Autodesk Inventor part; units mm, degrees
ref_plane "Płaszczyzna konstrukcyjna1" through (26, 10.6066, 10.6066) normal (0, 0.7071, 0.7071) x (-1, 0, 0)
ref_plane "Płaszczyzna konstrukcyjna2" through (26, 10.6066, -10.6066) normal (0, 0.7071, -0.7071) x (-1, 0, 0)
ref_plane "YZ Plane" through (0, 0, 0) normal (1, 0, 0) x (0, 1, 0)
sketch "Szkic1" plane through (0, 0, 0) normal (1, 0, 0) x (0, 1, 0)
  circle A0 centre (0, 0) radius 15
  dimension "d0" = 30
extrude "Wyciągnięcie proste1" add sketch "Szkic1" along normal blind 26
sketch "Szkic2" plane through (26, 0, 0) normal (1, 0, 0) x (0, 0, -1)
  point P0 (0, 0)
  point P1 (0, 0)
hole "Otwór1" at (26, 0, 0) direction (-1, 0, 0) diameter 8.5 end through all
sketch "Szkic3" plane through (26, 0, 0) normal (1, 0, 0) x (0, 0, -1)
  point P0 (0, 0)
  point P1 (11, 0)
  point P2 (0, 11)
  point P3 (-11, 0)
  point P4 (0, -11)
  dimension "d10" = 11
  dimension "d13" = 360
hole "Otwór2" at (26, 0, -11) at (26, 11, 0) at (26, 0, 11) at (26, -11, 0) direction (-1, 0, 0) diameter 3.5 depth 26 tip angle 118
sketch "Szkic4" plane through (26, 0, 0) normal (1, 0, 0) x (0, 0, -1)
  line L0 (0, 0) -> (-10.6066, 10.6066)
  line L1 (0, 0) -> (15, 0) construction
  line L2 (0, 0) -> (10.6066, 10.6066)
  line L3 (0, 0) -> (15, 0) construction
  dimension "d22" = 15
  dimension "d23" = 135
  dimension "d24" = 15
  dimension "d25" = 45
ref_plane "Płaszczyzna konstrukcyjna1" through (26, 10.6066, 10.6066) normal (0, 0.7071, 0.7071) x (-1, 0, 0)
ref_plane "Płaszczyzna konstrukcyjna2" through (26, 10.6066, -10.6066) normal (0, 0.7071, -0.7071) x (-1, 0, 0)
sketch "Szkic7" plane through (0, 0, 0) normal (-1, 0, 0) x (0, 0, 1)
  circle A0 centre (0, 0) radius 6.5
  dimension "d42" = 13
extrude "Wyciągnięcie proste2" cut sketch "Szkic7" against normal blind 5
sketch "Szkic13" plane through (5, 0, 0) normal (-1, 0, 0) x (0, 0, 1)
  circle A0 centre (0, 0) radius 5.5
  dimension "d80" = 11
extrude "Wyciągnięcie proste5" cut sketch "Szkic13" against normal blind 0.5
sketch "Szkic14" plane through (26, 0, 0) normal (1, 0, 0) x (0, 0, -1)
  circle A0 centre (0, 0) radius 6.5
  dimension "d83" = 13
extrude "Wyciągnięcie proste6" cut sketch "Szkic14" against normal blind 5
sketch "Szkic15" plane through (21, 0, 0) normal (1, 0, 0) x (0, 0, -1)
  circle A0 centre (0, 0) radius 5.5
  dimension "d86" = 11
extrude "Wyciągnięcie proste7" cut sketch "Szkic15" against normal blind 0.5
equation "\"d0\" = radius"
equation "\"d16\" = d1"
equation "\"d20\" = d1"
equation "\"d22\" = 0.5 * radius"
equation "\"d24\" = d22"
equation "\"radius\" = 30"
properties part number "piasta_kola_przedniego_fi8" material "Aluminum 6061"
Work out the finished part from the listing and answer in its coordinate system (mm). A direction names the side the tool comes from. Round coordinates to 2 decimals unless told otherwise and drop trailing zeros. Write each loop counter-clockwise with the first axis right and the second up, starting at its lowest first coordinate (ties: lowest second). Pieces come first, ordered by that corner, then holes. Notation, with made-up numbers: (2, -36.5) -> (28, -36.5) arc R5 ccw to (28, -29.5) -> close; hole circle Ø8 at (-27, -31). An arc over 180 degrees is marked (long way). Write each question's results on one line, items separated by ' | '.
Q1. Determine the mould class of faces 1 (the cylindrical face through (2.465, -3.955, -5.158)), 2 (the flat face through (0, 6, -3)), 3 (the cylindrical face through (12.818, -14.985, -0.66)), 4 (the cylindrical face through (20.75, -5.37, 1.19)) for opening direction Y: released by +Y, released by -Y, zero draft, split by the parting line, or undercut.
Data:
face 1: undercut | face 2: zero draft | face 3: split by the parting line | face 4: undercut
Q2. Section D-D, the plane x = 6.75 is taken. Write down the section's boundary in (y, z).
Data:
outline: circle Ø30 at (0, 0); hole circle Ø3.5 at (-11, 0); hole circle Ø8.5 at (0, 0); hole circle Ø3.5 at (0, -11); hole circle Ø3.5 at (0, 11); hole circle Ø3.5 at (11, 0)
Q3. Section C-C, the plane y = 11 is taken. Write down the section's boundary in (x, z).
Data:
outline: (0, -10.2) -> (26, -10.2) -> (26, -1.75) -> (0, -1.75) -> close; (0, 1.75) -> (26, 1.75) -> (26, 10.2) -> (0, 10.2) -> close
Q4. Flat-ended cylindrical pins translate along their axes: P1, Ø9, axis at y = 0, z = 0, coming from the -X side; P2, Ø10, axis at x = 7, z = -11.5, coming from the +Y side; P3, Ø12, axis at x = 20, z = 8.5, coming from the +Y side. Find the tip coordinate at first contact, or state that the pin passes through.
Data:
P1: x = 5.5 | P2: y = 13.52 | P3: y = 14.79
Q5. Which of the six approach directions +Z, -Z, +X, -X, +Y, -Y give full straight-line access (tool end or side, diameter ignored) to faces 5 (the cylindrical face through (23.535, -3.955, 5.158)), 6 (the cylindrical face through (5.25, -5.37, -1.19)), 7 (the cylindrical face through (12.895, -3.584, -2.285))?
Data:
face 5: +X | face 6: -X | face 7: +X, -X
Q6. Straight lines are drawn through the part: line 1 along Z through (x, y) = (2.25, 2.25); line 2 along Y through (x, z) = (11.5, -10.75); line 3 along Z through (x, y) = (3.5, -2). For each, find the intervals that lie inside material, in ascending order. Write a range as [from, to].
Data:
line 1: [-14.83, -6.1], [6.1, 14.83] | line 2: [-10.46, -1.73], [1.73, 10.46] | line 3: [-14.87, -6.18], [6.18, 14.87]
Q7. Section A-A, the plane z = 0 is taken. Give the number of separate pieces and of enclosed holes in the cut face, then the cut area to 4 significant figures.
Data:
separate pieces: 4 | enclosed holes: 0 | area: 329.5 mm^2
